Geometry: final body of the model. Coordinates: model frame, mm. A direction names the side the tool comes from. Give positions to 0.01 mm unless a question says otherwise; leave off trailing zeros. Loops run counter-clockwise (first coordinate to the right, second up) from the corner with the lowest first, then second, coordinate; pieces in that order, holes last.
Autodesk Inventor part; units mm, degrees
ref_plane "YZ Plane" through (0, 0, 0) normal (1, 0, 0) x (0, 1, 0)
ref_plane "XZ Plane" through (0, 0, 0) normal (0, 1, 0) x (-1, 0, 0)
ref_plane "XY Plane" through (0, 0, 0) normal (0, 0, 1) x (1, 0, 0)
sketch "Sketch1" plane through (0, 0, 0) normal (0, 1, 0) x (-1, 0, 0)
  line L0 (-38.1, 88.708) -> (38.1, 88.708)
  line L1 (38.1, 88.708) -> (38.1, -88.708)
  line L2 (38.1, -88.708) -> (-38.1, -88.708)
  line L3 (-38.1, -88.708) -> (-38.1, 88.708)
  line L4 (-38.1, 88.708) -> (38.1, -88.708) construction
  line L5 (38.1, 88.708) -> (-38.1, -88.708) construction
  point P0 (0, 0)
  dimension "d0" = 76.2
extrude "Extrusion1" add sketch "Sketch1" along normal blind 6.35
sketch "Sketch2" plane through (0, 6.35, 0) normal (0, 1, 0) x (1, 0, 0)
  line L0 (38.1, -88.708) -> (38.1, 88.708)
  line L1 (-38.1, -6.787) -> (38.1, -6.787)
  line L2 (38.1, -6.787) -> (38.1, 6.787)
  line L3 (38.1, 6.787) -> (-38.1, 6.787)
  line L4 (-38.1, 6.787) -> (-38.1, -6.787)
  line L5 (-38.1, -6.787) -> (38.1, 6.787) construction
  line L6 (38.1, -6.787) -> (-38.1, 6.787) construction
  line L7 (-38.1, 88.708) -> (38.1, 88.708)
  line L8 (38.1, 88.708) -> (38.1, 82.0757)
  line L9 (38.1, 82.0757) -> (-38.1, 82.0757)
  line L10 (-38.1, 82.0757) -> (-38.1, 88.708)
  point P0 (0, 0)
extrude "Extrusion2" add sketch "Sketch2" along normal blind 76.2
sketch "Sketch3" plane through (0, 6.35, 0) normal (0, 1, 0) x (1, 0, 0)
  line L0 (-38.1, -88.708) -> (-38.1, 88.708)
  line L1 (38.1, 88.708) -> (-38.1, 88.708)
  line L2 (-38.1, 88.708) -> (-38.1, 70.9931)
  line L3 (-38.1, 70.9931) -> (38.1, 70.9931)
  line L4 (38.1, 70.9931) -> (38.1, 88.708)
  point P0 (0, 0)
extrude "Extrusion3" add sketch "Sketch3" along normal blind 12.7
sketch "Sketch4" plane through (-38.1, 6.35, 6.787) normal (0, 0, 1) x (1, 0, 0)
  circle A0 centre (38.1, 42.2042) radius 6.35
  point P0 (38.1, -6.35)
  dimension "d7" = 12.7
extrude "Extrusion4" cut sketch "Sketch4" against normal blind 100.0125
sketch "Sketch5" plane through (-38.1, 6.35, 6.787) normal (0, 0, 1) x (1, 0, 0)
  circle A0 centre (38.1, 42.2042) radius 24.7775
  circle A1 centre (38.1, 42.2042) radius 6.35
  point P0 (38.1, -6.35)
extrude "Extrusion5" add sketch "Sketch5" along normal blind 57.15 contours A0 | A1
fillet "Fillet1" radius 6.35 1 edges at (-24.7775, 48.5542, 63.937)
sketch "Sketch6" plane through (0, 6.35, 0) normal (0, 1, 0) x (1, 0, 0)
  circle A0 centre (-26.2107, -78.7534) radius 5.2502
  circle A1 centre (-26.2107, 31.9702) radius 5.2572
  point P0 (0, 0)
extrude "Extrusion6" cut sketch "Sketch6" against normal blind 25.4
mirror "Mirror1" about plane through (0, 0, 0) normal (1, 0, 0) of "Extrusion6"
sketch "Sketch7" plane through (38.1, 6.35, -6.787) normal (0, 0, -1) x (-1, 0, 0)
  circle A0 centre (22.9263, 42.0163) radius 3.3075
  point P0 (38.1, -6.35)
extrude "Extrusion7" cut sketch "Sketch7" against normal blind 25.4
mirror "Mirror2" about plane through (0, 0, 0) normal (1, 0, 0) of "Extrusion7"
sketch "Sketch8" plane through (0, 6.35, 0) normal (0, 1, 0) x (1, 0, 0)
  point P0 (0, 0)
properties part number "Motor Fixture"
Item 1: Set-up query: faces 4 (the face through (-5.371, 72.743, 31.831)), 5 (the face through (0, 49, 63.937)), 6 (the face through (-13.65, 51.3, 5.74)). Return all of +Z, -Z, +X, -X, +Y, -Y with unobstructed straight access to the full face (end or side cutting, diameter ignored); none if empty.
Values follow:
face 4: +Z
face 5: +Z, +X, -X, +Y
face 6: none
Item 2: Draft query along Y for faces 1 (the face through (38.1, 26, -6)), 2 (the face through (1, 0, 1)), 3 (the face through (15, 48, 18.613)). Return one class per face: +Y half, -Y half, draft (parallel to the pull), parting line (faces both ways), or undercut.
Values follow:
face 1: draft
face 2: -Y half
face 3: undercut
Item 3: Pin query (flat end, axial travel): pin 1 (19.5 mm diameter, centred on x = -18, z = -45, fed in from +Y); pin 2 (9 mm diameter, centred on x = 14.5, z = -76.5, fed in from +Y); pin 3 (10 mm diameter, centred on x = -5, y = 12.5, fed in from +Z); pin 4 (6.5 mm diameter, centred on x = 26.21, z = 78.75, fed in from +Y). Return the tip coordinate at first contact, or that it passes through.
Values follow:
pin 1: stops at y = 6.35
pin 2: stops at y = 19.05
pin 3: stops at z = 6.79
pin 4: passes through
Item 4: Section query A-A on x = 0. Return loops of the section in (y, z), plus the area to 3 significant figures.
Values follow:
outline: (0, -88.71) - (42.2, -88.71) - (42.2, -82.08) - (19.05, -82.08) - (19.05, -70.99) - (6.35, -70.99) - (6.35, -6.79) - (42.2, -6.79) - (42.2, 6.79) - (54.9, 6.79) - (54.9, -6.79) - (82.55, -6.79) - (82.55, 6.79) - (73.33, 6.79) - (73.33, 57.59) arc R6.35 ccw to (66.98, 63.94) - (30.13, 63.94) arc R6.35 ccw to (23.78, 57.59) - (23.78, 6.79) - (6.35, 6.79) - (6.35, 88.71) - (0, 88.71) - close; (54.9, -88.71) - (82.55, -88.71) - (82.55, -82.08) - (54.9, -82.08) - close
area: 5,370 mm2
Item 5: Ray query, probe 1 along Z at (x, y) = (-28, 13.5); probe 2 along Z at (x, y) = (8.5, 53.5); probe 3 along Y at (x, z) = (0, -2). Return the intervals inside material, ascending.
Values follow:
probe 1: z = -88.71 to -70.99, -6.79 to 6.79
probe 2: z = -88.71 to -82.08, -6.79 to 63.94
probe 3: y = 0 to 42.2, 54.9 to 82.55
Item 6: Section query C-C on z = -77.5. Return loops of the section in (x, y).
Values follow:
outline: (-38.1, 0) - (38.1, 0) - (38.1, 19.05) - (-38.1, 19.05) - close
